Verification items for the finished model (mm, model axes). Face numbers are marked on the shaded views. A direction names the side the tool comes from. Give positions to 0.01 mm unless a question says otherwise; leave off trailing zeros. Order: outer loops, then holes, each group sorted by start corner. A loop starts at its lowest first (then second) coordinate and runs counter-clockwise, first axis right, second up.
(1) Mould release check, pull along X, two halves, no side actions. Record for the marked faces 3, 4 and 5: pulls with the +X half, pulls with the -X half, needs draft (parallel to the pull), parting line crosses it, or undercut.
(2) Sectioned sample at C-C on x = 92.5. Record the cut outline in (y, z).
(3) Gauge pin test, flat ends, axial feed: pin 1 (12 mm diameter, centred on y = 99.5, z = -69.5, fed in from +X); pin 2 (6 mm diameter, centred on y = 44.5, z = -88.5, fed in from -X); pin 3 (6 mm diameter, centred on x = 137, z = -36.5, fed in from -Y). Record the tip position at first contact, or that the pin passes through.
(4) Sectioned sample at D-D on z = -90.5. Record the cut outline in (x, y).
(5) Scan lines: L1, parallel to Y at x = 62.5, z = -142; L2, parallel to Z at x = 74, y = 27.5; L3, parallel to X at y = 25, z = -26. Record each from-to range of solid material in increasing order.
(6) Sectioned sample at A-A on y = 73.5. Record the cut outline in (x, z), plus the area to 3 significant figures.
(7) Access from +Z, -Z, +X, -X, +Y, -Y to the whole of each face (thin tool, end or side, straight path). Record for the marked faces 1 and 2.
(8) Sectioned sample at B-B on z = -120.5. Record the cut outline in (x, y).
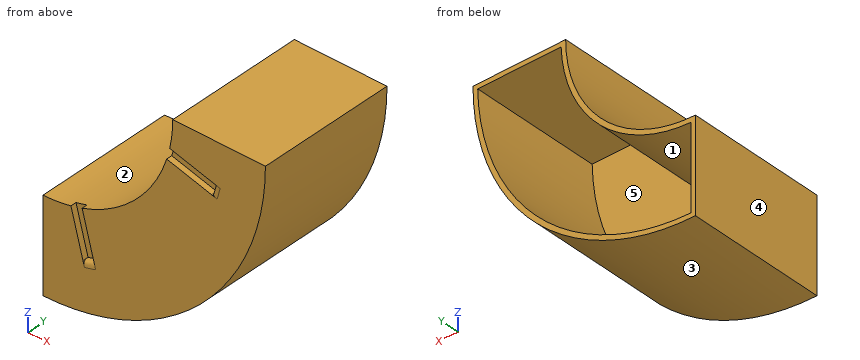
```python
from build123d import *

# Parameters (mm, degrees)
ESTRUSIONE_ESTRUSIONE1_DEPTH = 120
TAGLIO_ESTRUSIONE1_DEPTH     = 113
TAGLIO_ESTRUSIONE2_DEPTH     = 5
RACCORDO1_SIZE               = 5


with BuildPart() as part:
    # Schizzo1 → Estrusione-Estrusione1 (new body)
    with BuildSketch(Plane(origin=(0, 0, 0), x_dir=(1, 0, 0), z_dir=(0, 1, 0))):
        with BuildLine():
            Line((0, 112), (0, 192))
            ThreePointArc((0, 192), (135.764501988, 135.764501988), (192, 0))
            Line((192, 0), (112, 0))
            ThreePointArc((112, 0), (79.195959493, 79.195959493), (0, 112))
        make_face()
    extrude(amount=ESTRUSIONE_ESTRUSIONE1_DEPTH)

    # Schizzo2 → Taglio-Estrusione1 (cut)
    with BuildSketch(Plane(origin=(0, 120, 0), x_dir=(1, 0, 0), z_dir=(0, 1, 0))):
        with BuildLine():
            Line((4, 115.93101397), (4, 187.957441992))
            ThreePointArc((4, 187.957441992), (132.936074863, 132.936074863), (187.957441992, 4))
            Line((187.957441992, 4), (115.93101397, 4))
            ThreePointArc((115.93101397, 4), (82.024386618, 82.024386618), (4, 115.93101397))
        make_face()
    extrude(amount=-TAGLIO_ESTRUSIONE1_DEPTH, mode=Mode.SUBTRACT)

    # Schizzo3 → Taglio-Estrusione2 (cut)
    with BuildSketch(Plane.XZ):
        with BuildLine():
            Line((34.489575502, -148.035364632), (24.129203459, -109.369929782))
            ThreePointArc((24.129203459, -109.369929782), (28.987733051, -108.183692544), (33.788461722, -106.781739331))
            Line((33.788461722, -106.781739331), (44.148833765, -145.447174181))
            ThreePointArc((44.148833765, -145.447174181), (39.340494856, -146.820725596), (34.489575502, -148.035364632))
        make_face()
        with BuildLine():
            Line((145.447174181, -44.148833765), (106.781739331, -33.788461722))
            ThreePointArc((106.781739331, -33.788461722), (108.183692544, -28.987733051), (109.369929782, -24.129203459))
            Line((109.369929782, -24.129203459), (148.035364632, -34.489575502))
            ThreePointArc((148.035364632, -34.489575502), (146.820725596, -39.340494856), (145.447174181, -44.148833765))
        make_face()
    extrude(amount=-TAGLIO_ESTRUSIONE2_DEPTH, mode=Mode.SUBTRACT)

    # Raccordo1
    # a fillet whose section is not a circle: 5 mm, written as the material it takes off along each edge
    with BuildSketch(Plane(origin=(0, 0, 0), x_dir=(0.9892644198784365, 0, -0.14613660582681076), z_dir=(0.14613660582681076, 0, 0.9892644198784365))) as raccordo1_piece_1_section:
        with BuildLine():
            Bezier((152 + RACCORDO1_SIZE, 0), (152, 0), (152, RACCORDO1_SIZE), weights=[1, 1.5, 1])
            Line((152, RACCORDO1_SIZE), (152, 0))
            Line((152, 0), (152 + RACCORDO1_SIZE, 0))
        make_face()
    raccordo1_piece_1 = revolve(axis=Axis((0, 0, 0), (0, 1, 0)), revolution_arc=13.193793896, mode=Mode.PRIVATE)
    raccordo1_piece_1 = split(raccordo1_piece_1, bisect_by=Plane(origin=(-1.294095226, 0, -4.829629131), z_dir=(0.2588190451025214, 0, 0.9659258262890682)), keep=Keep.TOP, mode=Mode.PRIVATE)
    raccordo1_piece_1 = split(raccordo1_piece_1, bisect_by=Plane(origin=(1.294095225, 0, 4.829629131), z_dir=(-0.25881904510252096, 0, -0.9659258262890682)), keep=Keep.TOP, mode=Mode.PRIVATE)
    add(raccordo1_piece_1, mode=Mode.SUBTRACT)
    with BuildSketch(Plane(origin=(0, 0, 0), x_dir=(0.36807419687030923, 0, -0.9297964215882295), z_dir=(0.9297964215882295, 0, 0.36807419687030923))) as raccordo1_piece_2_section:
        with BuildLine():
            Bezier((152 + RACCORDO1_SIZE, 0), (152, 0), (152, RACCORDO1_SIZE), weights=[1, 1.5, 1])
            Line((152, RACCORDO1_SIZE), (152, 0))
            Line((152, 0), (152 + RACCORDO1_SIZE, 0))
        make_face()
    raccordo1_piece_2 = revolve(axis=Axis((0, 0, 0), (0, 1, 0)), revolution_arc=13.193793896, mode=Mode.PRIVATE)
    raccordo1_piece_2 = split(raccordo1_piece_2, bisect_by=Plane(origin=(-4.829629131, 0, -1.294095225), z_dir=(0.965925826289068, 0, 0.2588190451025222)), keep=Keep.TOP, mode=Mode.PRIVATE)
    raccordo1_piece_2 = split(raccordo1_piece_2, bisect_by=Plane(origin=(4.829629131, 0, 1.294095226), z_dir=(-0.965925826289068, 0, -0.2588190451025218)), keep=Keep.TOP, mode=Mode.PRIVATE)
    add(raccordo1_piece_2, mode=Mode.SUBTRACT)


solid = part.part
```
Ans:
1. face 3: pulls with the +X half
1. face 4: pulls with the -X half
1. face 5: undercut
2. outline: (0, -168.25) - (120, -168.25) - (120, -163.67) - (7, -163.67) - (7, -70) - (120, -70) - (120, -63.15) - (0, -63.15) - close
3. pin 1: stops at x = 181.2
3. pin 2: stops at x = 64.59
3. pin 3: stops at y = 5
4. outline: (65.98, 0) - (169.33, 0) - (169.33, 120) - (164.78, 120) - (164.78, 7) - (72.57, 7) - (72.57, 120) - (65.98, 120) - close
5. L1: y = 0 to 7
5. L2: z = -177.17 to -172.82, -89.33 to -84.07
5. L3: x = 108.94 to 113.05, 186.19 to 190.23
6. outline: (0, -192) arc R192 ccw to (192, 0) - (112, 0) arc R112 cw to (0, -112) - close; hole (4, -187.96) arc R188 ccw to (187.96, -4) - (115.93, -4) arc R116 cw to (4, -115.93) - close
6. area: 2,490 mm2
7. face 1: +Y
7. face 2: +Z, -X, +Y, -Y
8. outline: (0, 0) - (27.11, 0) - (27.11, 5) - (37.46, 5) - (37.46, 0) - (149.48, 0) - (149.48, 120) - (144.3, 120) - (144.3, 7) - (4, 7) - (4, 120) - (0, 120) - close
